Autodesk Inventor part; units mm, degrees
ref_plane "YZ Plane" through (0, 0, 0) normal (1, 0, 0) x (0, 1, 0)
ref_plane "XZ Plane" through (0, 0, 0) normal (0, 1, 0) x (-1, 0, 0)
ref_plane "XY Plane" through (0, 0, 0) normal (0, 0, 1) x (1, 0, 0)
sketch "Skizze1" plane through (0, 0, 0) normal (0, 1, 0) x (-1, 0, 0)
  line L0 (-5, 0) -> (-5, -3)
  line L1 (-5, -3) -> (0, -3)
  line L2 (-5, 0) -> (-10, 0)
  line L3 (-10, 0) -> (-10, -3)
  line L4 (-10, -3) -> (-15, -3)
  line L5 (-15, 0) -> (-15, -3)
  line L6 (-15, 0) -> (-20, 0)
  line L7 (-20, 0) -> (-20, -3)
  line L8 (-20, -3) -> (-25, -3)
  line L9 (-25, 0) -> (-25, -3)
  line L10 (-25, 0) -> (-30, 0)
  line L11 (-30, 0) -> (-30, -3)
  line L12 (-30, -3) -> (-35, -3)
  line L13 (-35, 0) -> (-35, -3)
  line L14 (-35, 0) -> (-40, 0)
  line L15 (-40, 0) -> (-40, -3)
  line L16 (-40, -3) -> (-45, -3)
  line L17 (-45, 0) -> (-45, -3)
  line L18 (-45, 0) -> (-50, 0)
  line L19 (-50, 0) -> (-50, -3)
  line L20 (-50, -3) -> (-55, -3)
  line L21 (-55, -3) -> (-55, -8)
  line L22 (-55, -8) -> (-52, -8)
  line L23 (-52, -8) -> (-52, -13)
  line L24 (-52, -13) -> (-55, -13)
  line L25 (0, -3) -> (0, -8)
  line L26 (0, -8) -> (-3, -8)
  line L27 (-3, -8) -> (-3, -13)
  line L28 (-3, -13) -> (0, -13)
  line L29 (-52, -18) -> (-52, -23)
  line L30 (-55, -13) -> (-55, -18)
  line L31 (-52, -23) -> (-55, -23)
  line L32 (-55, -18) -> (-52, -18)
  line L33 (-3, -18) -> (-3, -23)
  line L34 (-3, -23) -> (0, -23)
  line L35 (0, -18) -> (-3, -18)
  line L36 (0, -13) -> (0, -18)
  line L37 (0, -38) -> (-5, -38)
  line L38 (-5, -38) -> (-5, -35)
  line L39 (-5, -35) -> (-10, -35)
  line L40 (-10, -35) -> (-10, -38)
  line L41 (-15, -35) -> (-20, -35)
  line L42 (-20, -35) -> (-20, -38)
  line L43 (-10, -38) -> (-15, -38)
  line L44 (-15, -38) -> (-15, -35)
  line L45 (-25, -35) -> (-30, -35)
  line L46 (-30, -35) -> (-30, -38)
  line L47 (-20, -38) -> (-25, -38)
  line L48 (-25, -38) -> (-25, -35)
  line L49 (-35, -35) -> (-40, -35)
  line L50 (-40, -35) -> (-40, -38)
  line L51 (-30, -38) -> (-35, -38)
  line L52 (-35, -38) -> (-35, -35)
  line L53 (-45, -35) -> (-50, -35)
  line L54 (-50, -35) -> (-50, -38)
  line L55 (-40, -38) -> (-45, -38)
  line L56 (-45, -38) -> (-45, -35)
  line L57 (-50, -38) -> (-55, -38)
  line L58 (-35.75, -24) -> (-43.75, -24)
  line L59 (-44.75, -23) -> (-44.75, -15)
  line L60 (-43.75, -14) -> (-35.75, -14)
  line L61 (-34.75, -15) -> (-34.75, -23)
  arc A0 (-35.75, -24) -> (-34.75, -23) centre (-35.75, -23) ccw
  arc A1 (-44.75, -23) -> (-43.75, -24) centre (-43.75, -23) ccw
  arc A2 (-43.75, -14) -> (-44.75, -15) centre (-43.75, -15) ccw
  arc A3 (-34.75, -15) -> (-35.75, -14) centre (-35.75, -15) ccw
  line L62 (-27.5, -38) -> (-27.5, 0) construction
  line L63 (-27.5, -19) -> (-52, -19) construction
  line L64 (-52, -28) -> (-52, -33)
  line L65 (-55, -23) -> (-55, -28)
  line L66 (-52, -33) -> (-55, -33)
  line L67 (-55, -28) -> (-52, -28)
  line L68 (-3, -28) -> (-3, -33)
  line L69 (-3, -33) -> (0, -33)
  line L70 (0, -28) -> (-3, -28)
  line L71 (0, -23) -> (0, -28)
  line L72 (0, -38) -> (0, -33)
  line L73 (-55, -33) -> (-55, -38)
  point P0 (0, 0)
  point P1 (-34.75, -19)
  point P2 (-39.75, -19)
  point P3 (-39.75, -24)
  dimension "d2" = 5
  dimension "d3" = 3
  dimension "d6" = 10
  dimension "d22" = 10
  dimension "d29" = 10
  dimension "d34" = 1
  dimension "d36" = 10
  dimension "d37" = 10
extrude "Extrusion1" add sketch "Skizze1" along normal blind 3
properties part number "plate_front_small" material "Holz (Kirsche)"
Part model, mm, in its own coordinate system. A direction names the side the tool comes from. Round coordinates to 2 decimals unless told otherwise and drop trailing zeros. Order: outer loops, then holes, each group sorted by start corner. A loop starts at its lowest first (then second) coordinate and runs counter-clockwise, first axis right, second up. Notation, with made-up numbers: M -5.75,-27.5 L 49.25,-27.5 A21 ccw 49.25,10.5 Z; hole C 38.25,44 d11. An arc over 180 degrees is marked long. Put each result on its own line as item: value. Start each with the question number.
1. Tool access for faces 4 (the face through (12, 1, -3)), 5 (the face through (50, 1, -1)), 6 (the face through (3, 1, -3)), 7 (the face through (15, 1, -37)): list every direction of +Z, -Z, +X, -X, +Y, -Y with a clear straight run to the whole face (end or side of a thin tool).
2. Slice it at C-C on x = 14. List the corners of the cut face in (y, z).
3. Slice it at A-A on x = 42. List the corners of the cut face in (y, z), then the cut area to 3 significant figures.
4. Two-plate mould, pull along X, no slides. Class faces 1 (the face through (53, 1, -23)), 2 (the face through (17, 1, -35)), 3 (the face through (55, 1, -35)): +X half, -X half, draft (parallel to the pull), parting line (faces both ways), or undercut.
5. Drop flat-ended pins along their axis: pin 1 (1.5 mm diameter, centred on x = 22.5, y = 1.5, fed in from +Z); pin 2 (0.9 mm diameter, centred on y = 2, z = -1.5, fed in from -X); pin 3 (0.9 mm diameter, centred on y = 2, z = -10, fed in from +X). Give the stop position or say it passes through.
6. Drill centre lines: probe 1 along X at (y, z) = (2, -2); probe 2 along X at (y, z) = (2.25, -21.5); probe 3 along Z at (x, y) = (39, 2.2). Where is each one in solid material? Low to high. Write a range as [from, to].
7. Slice it at B-B on z = -30.5. List the corners of the cut face in (x, y).
Findings:
1. face 4: +Z, +Y, -Y
1. face 5: +Z, +X, +Y, -Y
1. face 6: +Z, -X, +Y, -Y
1. face 7: -Z, +Y, -Y
2. outline: M 0,-38 L 3,-38 L 3,-3 L 0,-3 Z
3. outline: M 0,-38 L 3,-38 L 3,-24 L 0,-24 Z; M 0,-14 L 3,-14 L 3,-3 L 0,-3 Z
3. area: 75.0 mm2
4. face 1: draft
4. face 2: undercut
4. face 3: +X half
5. pin 1: z = -3
5. pin 2: x = 5
5. pin 3: x = 52
6. probe 1: [5, 10], [15, 20], [25, 30], [35, 40], [45, 50]
6. probe 2: [3, 34.75], [44.75, 52]
6. probe 3: [-35, -24], [-14, 0]
7. outline: M 3,0 L 52,0 L 52,3 L 3,3 Z
